```python
from build123d import *

# Parameters (mm, degrees)
SKETCH1_R                 = 2.85
SKETCH1_R_2               = 2
BOSS_EXTRUDE1_DEPTH       = 59
SKETCH1_4_R               = 2
BOSS_EXTRUDE2_DEPTH       = 7
M4X0_7_TAPPED_HOLE1_D     = 3.3
M4X0_7_TAPPED_HOLE1_DEPTH = 10.1
M4X0_7_TAPPED_HOLE1_TIP   = 0.991420021
CHAMFER1_SIZE             = 0.5


with BuildPart() as part:
    # Sketch1 → Boss-Extrude1 (new body)
    with BuildSketch(Plane(origin=(0, 0, 0), x_dir=(1, 0, 0), z_dir=(0, 1, 0))):
        with Locations(Location((0, 0, 0), (0, 0, 270))):
            Circle(SKETCH1_R)
        Circle(SKETCH1_R_2, mode=Mode.SUBTRACT)
        Circle(SKETCH1_R_2)
    extrude(amount=BOSS_EXTRUDE1_DEPTH)

    # Sketch1_4 → Boss-Extrude2 (add)
    with BuildSketch(Plane(origin=(0, 0, 0), x_dir=(1, 0, 0), z_dir=(0, 1, 0))):
        with Locations(Location((0, 0, 0), (0, 0, 270))):
            Circle(SKETCH1_4_R)
    extrude(amount=-BOSS_EXTRUDE2_DEPTH)

    # M4x0.7 Tapped Hole1
    with Locations(Plane(origin=(0, 59, 0), x_dir=(1, 0, 0), z_dir=(0, 1, 0))):
        with Locations((0, 0)):
            Hole(M4X0_7_TAPPED_HOLE1_D / 2, depth=M4X0_7_TAPPED_HOLE1_DEPTH)
            with Locations((0, 0, -(M4X0_7_TAPPED_HOLE1_DEPTH + M4X0_7_TAPPED_HOLE1_TIP / 2))):  # 118° drill point
                Cone(0, M4X0_7_TAPPED_HOLE1_D / 2, M4X0_7_TAPPED_HOLE1_TIP, mode=Mode.SUBTRACT)

    # Chamfer1
    chamfer1_edges = [part.edges().sort_by_distance(p)[0] for p in [
        (0, -7, -2),
    ]]
    chamfer(chamfer1_edges, length=CHAMFER1_SIZE)


solid = part.part
```
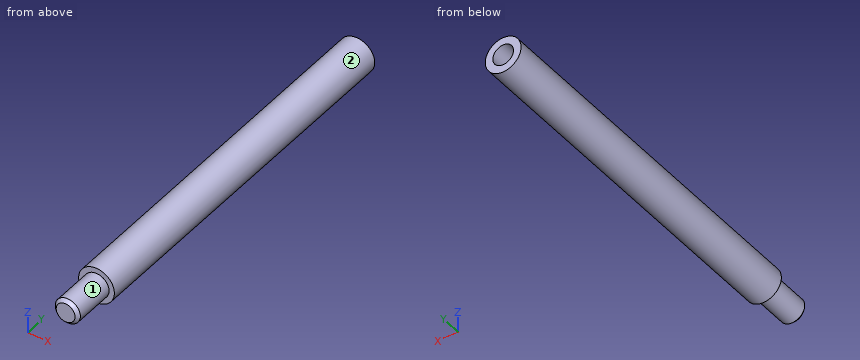
Can you work these out from the model? Positions are in its coordinate system, mm. Face numbers are marked on the shaded views. A direction names the side the tool comes from. Round coordinates to 2 decimals unless told otherwise and drop trailing zeros. Loops run counter-clockwise (first coordinate to the right, second up) from the corner with the lowest first, then second, coordinate; pieces in that order, holes last.
Item 1: Which directions (+Z, -Z, +X, -X, +Y, -Y) give clear straight access to the entire face, cutting with the end or side of a thin tool? Please do the marked faces 1 and 2.
Item 2: Suppose I cut it at B-B, the plane y = 51. Write out the boundary of the cut face in (x, z), then the cut area to 3 significant figures.
Item 3: Suppose I cut it at A-A, the plane y = -2.5. Write out the boundary of the cut face in (x, z), then the cut area to 3 significant figures.
Item 4: Suppose I cut it at C-C, the plane y = 22. Write out the boundary of the cut face in (x, z), then the cut area to 3 significant figures.
Item 5: Will these pins go through, and if not, where does the flat tip stop? pin 1 Ø1.5 at (x, y) = (-1.5, 12.5) entering from -Z; pin 2 Ø3 at (x, z) = (0, 0) entering from +Y.
Item 6: Please list where these lines run through material, in increasing order: L1, parallel to Y at x = -0.7, z = -2.15; L2, parallel to X at y = 52, z = -0.15; L3, parallel to Y at x = 1.65, z = -0.4.
Reported:
1. face 1: -Y
1. face 2: +Y, -Y
2. outline: circle Ø5.7 at (0, 0); hole circle Ø3.3 at (0, 0)
2. area: 17.0 mm2
3. outline: circle Ø4 at (0, 0)
3. area: 12.6 mm2
4. outline: circle Ø5.7 at (0, 0)
4. area: 25.5 mm2
5. pin 1: stops at z = -2.75
5. pin 2: stops at y = 48.81
6. L1: y = 0 to 59
6. L2: x = -2.85 to -1.64, 1.64 to 2.85
6. L3: y = -6.8 to 59
